Geometry: final body of the model. Coordinates: model frame, mm. A direction names the side the tool comes from. Give positions to 0.01 mm unless a question says otherwise; leave off trailing zeros. Loops run counter-clockwise (first coordinate to the right, second up) from the corner with the lowest first, then second, coordinate; pieces in that order, holes last. Notation, with made-up numbers: (61.5, 35) - (79.5, 35) arc R19 ccw to (79.5, 47) - close; hole circle Ø10 at (58, 89.5). An arc over 180 degrees is marked (long way). Answer in a Markdown table with one row per item.
from build123d import *

# Parameters (mm, degrees)
SKETCH_1_R               = 5
EXTRUDE_1_DEPTH          = 83
SKETCH_3_R               = 9
EXTRUDE_2_DEPTH          = 4
SKETCH_4_R               = 6
EXTRUDE_3_DEPTH          = 22
CUT_EXTRUDE_1_DEPTH      = 110.740603242
CUT_EXTRUDE_1_DEPTH_BACK = 110.740603242
SKETCH_5_R               = 2
CHAMFER_1_SIZE           = 1


# Read off the part's stored shape, not the designer's step: M10 机械螺纹 螺柱1
with BuildPart() as part:
    # 草图1 → 凸台-拉伸1 (new body)
    with BuildSketch(Plane.XY):
        Circle(SKETCH_1_R)
    extrude(amount=-EXTRUDE_1_DEPTH)

    # M10 机械螺纹 螺柱1 outline → M10 机械螺纹 螺柱1 (revolve, cut)
    with BuildSketch(Plane.XZ):
        Polygon((5, 0), (4.188, 0), (5, -0.812), align=None)
    revolve(axis=Axis((0, 0, 0), (0, 0, 1)), mode=Mode.SUBTRACT)

    # 草图3 → 凸台-拉伸2 (add)
    with BuildSketch(Plane(origin=(0, 0, -83), x_dir=(-1, 0, 0), z_dir=(0, 0, -1))):
        Circle(SKETCH_3_R)
    extrude(amount=EXTRUDE_2_DEPTH)

    # 草图4 → 凸台-拉伸3 (add)
    with BuildSketch(Plane(origin=(0, 0, -87), x_dir=(-1, 0, 0), z_dir=(0, 0, -1))):
        Circle(SKETCH_4_R)
    extrude(amount=EXTRUDE_3_DEPTH)

    # 草图5 → 切除-拉伸1 (cut, two sides: drawn at the far end of the back side and taken through both)
    with BuildSketch(Plane(origin=(0, 0, 0), x_dir=(1, 0, 0), z_dir=(0, 1, 0)).offset(-CUT_EXTRUDE_1_DEPTH_BACK)):
        with Locations(Location((0, 95, 0), (0, 0, 270))):
            Circle(SKETCH_5_R)
    extrude(amount=CUT_EXTRUDE_1_DEPTH + CUT_EXTRUDE_1_DEPTH_BACK, mode=Mode.SUBTRACT)

    # 倒角1
    chamfer_1_edges = [part.edges().sort_by_distance(p)[0] for p in [
        (6, 0, -109),
    ]]
    chamfer(chamfer_1_edges, length=CHAMFER_1_SIZE)


solid = part.part
Q1. Material intervals for line 1 along Z through (x, y) = (0, 1.75); line 2 along Z through (x, y) = (-7, -5.25); line 3 along X through (y, z) = (0.25, -75), sorted ascending.
Check values:
| item | result |
|---|---|
| line 1 | -109 to -97, -93 to 0 |
| line 2 | -87 to -83 |
| line 3 | -4.99 to 4.99 |
Q2. Cut plane B-B (y = 0). Output: boundary loops of the cut face in (x, z).
Check values:
| item | result |
|---|---|
| outline | (-9, -87) - (-6, -87) - (-6, -108) - (-5, -109) - (5, -109) - (6, -108) - (6, -87) - (9, -87) - (9, -83) - (5, -83) - (5, -0.81) - (4.19, 0) - (-4.19, 0) - (-5, -0.81) - (-5, -83) - (-9, -83) - close; hole circle Ø4 at (0, -95) |
Q3. First-contact query: pin 1 (1.5 mm diameter, centred on x = 1, y = -3, fed in from +Z); pin 2 (3 mm diameter, centred on x = 0, z = -95, fed in from -Y) (1 decimal); pin 3 (8 mm diameter, centred on x = -0.5, z = -96, fed in from -Y); pin 4 (2 mm diameter, centred on x = 2.5, z = -43.5, fed in from -Y). Flat tips, straight axial feed; report the tip coordinate or a pass-through.
Check values:
| item | result |
|---|---|
| pin 1 | z = 0 |
| pin 2 | through |
| pin 3 | y = -6 |
| pin 4 | y = -4.77 |
Q4. Cut plane C-C (z = -95). Output: boundary loops of the cut face in (x, y), and give its area (3 significant figures).
Check values:
| item | result |
|---|---|
| outline | (-2, -5.66) - (-2, 5.66) arc R6 ccw to start; (2, -5.66) arc R6 ccw to (2, 5.66) - close |
| area | 66.0 mm² |
Q5. Draft query along X for faces 1 (the flat face through (0, 0, 0)), 2 (the cylindrical face through (0.601, -0.084, -93.092)), 3 (the cylindrical face through (-5.54, -2.3, -97.35)). Return one class per face: pulls with the +X half, pulls with the -X half, needs draft (parallel to the pull), parting line crosses it, or undercut.
Check values:
| item | result |
|---|---|
| face 1 | needs draft |
| face 2 | undercut |
| face 3 | parting line crosses it |
Q6. Reachability of faces 4 (the flat face through (-2, -6, -87)), 5 (the cylindrical face through (1.172, 8.923, -84.972)), 6 (the flat face through (-4, -4, -83)) from +Z, -Z, +X, -X, +Y, -Y: full face, straight path, thin tool, end or side. Return the list, or none.
Check values:
| item | result |
|---|---|
| face 4 | -Z |
| face 5 | +Z, -Z |
| face 6 | +Z |
Q7. Cut plane D-D (z = -28). Output: boundary loops of the cut face in (x, y).
Check values:
| item | result |
|---|---|
| outline | circle Ø10 at (0, 0) |
Q8. Cut plane A-A (x = 0). Output: boundary loops of the cut face in (y, z), and give its area (3 significant figures).
Check values:
| item | result |
|---|---|
| outline | (-9, -87) - (-6, -87) - (-6, -93) - (6, -93) - (6, -87) - (9, -87) - (9, -83) - (5, -83) - (5, -0.81) - (4.19, 0) - (-4.19, 0) - (-5, -0.81) - (-5, -83) - (-9, -83) - close; (-6, -108) - (-5, -109) - (5, -109) - (6, -108) - (6, -97) - (-6, -97) - close |
| area | 1,120 mm² |
